from build123d import *

# Parameters (mm, degrees)
EXTRUDE_1_DEPTH          = 200
CUT_EXTRUDE_1_DEPTH      = 222.718927326
CUT_EXTRUDE_1_DEPTH_BACK = 222.718927326
SKETCH_2_R               = 150
SKETCH_2_R_2             = 1.5
EXTRUDE_4_DEPTH          = 11.25
EXTRUDE_4_DEPTH_BACK     = 11.25
SKETCH_5_R               = 1.5
CUT_EXTRUDE_2_DEPTH      = 133.789577673
CUT_EXTRUDE_2_DEPTH_BACK = 133.789577673


with BuildPart() as part:
    # Эскиз1 → Бобышка-Вытянуть1 (new body)
    with BuildSketch(Plane(origin=(0, 0, 0), x_dir=(1, 0, 0), z_dir=(0, 1, 0))):
        Polygon((-63.065580883, 65.518470958), (69.761111645, 65.518470958), (2.121320344, -2.121320344), (0, 0), (-2.121320344, -2.121320344), (-69.761111645, 65.518470958), align=None)
    extrude(amount=EXTRUDE_1_DEPTH)

    # Эскиз2 → Вырез-Вытянуть1 (cut, two sides: drawn at the far end of the back side and taken through both)
    with BuildSketch(Plane(origin=(0, 0, 0), x_dir=(0, 0, -1), z_dir=(1, 0, 0)).offset(-CUT_EXTRUDE_1_DEPTH_BACK)):
        with Locations((-2.121320344, 100)):
            Circle(SKETCH_2_R)
        with Locations((-2.121320344, 100)):
            Circle(SKETCH_2_R_2, mode=Mode.SUBTRACT)
        Polygon((27.212959944, 126.107382569), (27.212959944, 73.892617431), (-7.080612422, 86.374456999), (-2.121320344, 100), (-7.080612422, 113.625543001), align=None, mode=Mode.SUBTRACT)
    extrude(amount=CUT_EXTRUDE_1_DEPTH + CUT_EXTRUDE_1_DEPTH_BACK, mode=Mode.SUBTRACT)

    # Эскиз5 → Бобышка-Вытянуть4 (add, two sides: drawn at the far end of the back side and taken through both)
    with BuildSketch(Plane(origin=(0, 0, 0), x_dir=(0, 0, -1), z_dir=(1, 0, 0)).offset(-EXTRUDE_4_DEPTH_BACK)):
        with BuildLine():
            ThreePointArc((-6.364433098, 98.5), (2.379124729, 100), (-6.364433098, 101.5))
            Line((-6.364433098, 101.5), (-15.643969281, 101.5))
            Line((-15.643969281, 101.5), (-15.643969281, 98.5))
            Line((-15.643969281, 98.5), (-6.364433098, 98.5))
        make_face()
        with Locations((-2.121320344, 100)):
            Circle(SKETCH_5_R, mode=Mode.SUBTRACT)
    extrude(amount=EXTRUDE_4_DEPTH + EXTRUDE_4_DEPTH_BACK)

    # Эскиз6 → Вырез-Вытянуть2 (cut, two sides: drawn at the far end of the back side and taken through both)
    with BuildSketch(Plane(origin=(0, 0, 0), x_dir=(1, 0, 0), z_dir=(0, 1, 0)).offset(-CUT_EXTRUDE_2_DEPTH_BACK)):
        Polygon((-50.182829752, 24.037490431), (0, 24.037490431), (93.439383522, 24.037490431), (93.439383522, 164.04737871), (-160.316075238, 164.04737871), (-160.316075238, 24.037490431), align=None)
    extrude(amount=CUT_EXTRUDE_2_DEPTH + CUT_EXTRUDE_2_DEPTH_BACK, mode=Mode.SUBTRACT)


solid = part.part
Source: CAD feature listing. Evaluate the final solid. Frame: model axes, mm. A direction names the side the tool comes from. Round coordinates to 2 decimals unless told otherwise and drop trailing zeros. Loops run counter-clockwise (first coordinate to the right, second up) from the corner with the lowest first, then second, coordinate; pieces in that order, holes last. Notation, with made-up numbers: M 89.25,-30.75 L 111.25,-30.75 A10 ccw 111.25,-25.75 Z; hole C 73.25,26.25 d9. An arc over 180 degrees is marked long. Return JSON: item names as keys, results as strings. Group by question number.
1. Section query B-B on y = 100. Output: boundary loops of the cut face in (x, z).
2. Section query C-C on z = -1. Output: boundary loops of the cut face in (x, y), and give its area (3 significant figures).
3. Reachability of faces 1 (the face through (11.25, 100, 5)), 2 (the face through (0, 101.5, 11)), 3 (the face through (-0.158, 97.415, 5.805)) from +Z, -Z, +X, -X, +Y, -Y: full face, straight path, thin tool, end or side. Return the list, or none.
4. Section query A-A on x = -9.5. Output: boundary loops of the cut face in (y, z).
5. Mould query, pull axis Y, two halves, no side actions, for faces 4 (the face through (-11.25, 100, 5)), 5 (the face through (0, 98.5, 11)), 6 (the face through (2.715, 99.979, 1.527)). Classes: released by +Y, released by -Y, zero draft, split by the parting line, or undercut.
6. Section query D-D on y = 106.5. Output: boundary loops of the cut face in (x, z).
7. Material intervals for line 1 along Z through (x, y) = (-5, 100); line 2 along Z through (x, y) = (3, 100); line 3 along X through (y, z) = (100, 11), sorted ascending. Write a range as from..to.
8. Pin query (flat end, axial travel): pin 1 (7.5 mm diameter, centred on x = 4.5, z = 9, fed in from -Y) (3 decimals); pin 2 (2.5 mm diameter, centred on y = 101.5, z = 4.5, fed in from -X); pin 3 (5 mm diameter, centred on x = -21.5, y = 103, fed in from +Z). Return the tip coordinate at first contact, or that it passes through.
Checks:
{
 "1": {"outline": "M -28.28,-24.04 L 28.28,-24.04 L 6.62,-2.38 L 11.25,-2.38 L 11.25,0.62 L 3.62,0.62 L 2.12,2.12 L 0.62,0.62 L -0.62,0.62 L -2.12,2.12 L -3.62,0.62 L -11.25,0.62 L -11.25,-2.38 L -6.62,-2.38 Z; M -11.25,3.62 L 11.25,3.62 L 11.25,15.64 L -11.25,15.64 Z"},
 "2": {"outline": "M -11.25,96.76 L -5.24,96.76 L -5.24,83.43 L 5.24,83.43 L 5.24,96.76 L 11.25,96.76 L 11.25,103.24 L 5.24,103.24 L 5.24,116.57 L -5.24,116.57 L -5.24,103.24 L -11.25,103.24 Z", "area": "425 mm²"},
 "3": {"face 1": "+Z, +X, +Y, -Y", "face 2": "+Z, +X, -X, +Y", "face 3": "none"},
 "4": {"outline": "M 75.05,-24.04 L 124.95,-24.04 L 118.12,-5.26 L 81.88,-5.26 Z; M 98.5,6.36 A4.5 ccw long 101.5,6.36 L 101.5,15.64 L 98.5,15.64 Z; hole C 100,2.12 d3"},
 "5": {"face 4": "zero draft", "face 5": "released by -Y", "face 6": "undercut"},
 "6": {"outline": "M -28.28,-24.04 L 28.28,-24.04 L 2.12,2.12 L 0,0 L -2.12,2.12 Z"},
 "7": {"line 1": "z = -24.04..0.62, 3.62..15.64", "line 2": "z = -24.04..1.24, 3.62..15.64", "line 3": "x = -11.25..11.25"},
 "8": {"pin 1": "stops at y = 96.765", "pin 2": "stops at x = -11.25", "pin 3": "stops at z = -14.76"}
}
